from build123d import *

# Parameters (mm, degrees)
F1_DEPTH = 3


with BuildPart() as f1:
    # F0 (on Top) → F1 (new body)
    with BuildSketch(Plane.XY):
        with BuildLine():
            Line((-8, 15), (-0.625, 15))
            Line((-0.625, 15), (6.75, 15))
            Line((6.75, 15), (13.042543, 8.707457))
            Line((13.042543, 8.707457), (13.042543, 1.332457))
            Line((13.042543, 1.332457), (13.042543, -6.042543))
            Line((13.042543, -6.042543), (9.542543, -9.542543))
            ThreePointArc((9.542543, -9.542543), (8.864734, -11.345012), (9.773969, -13.042543))
            Line((9.773969, -13.042543), (14.542543, -13.042543))
            Line((14.542543, -13.042543), (14.542543, 16.5))
            Line((14.542543, 16.5), (-15, 16.5))
            Line((-15, 16.5), (-15, 11.5))
            ThreePointArc((-15, 11.5), (-13.25, 10.775126), (-11.5, 11.5))
            Line((-11.5, 11.5), (-8, 15))
        make_face()
    extrude(amount=F1_DEPTH)


solid = f1.part
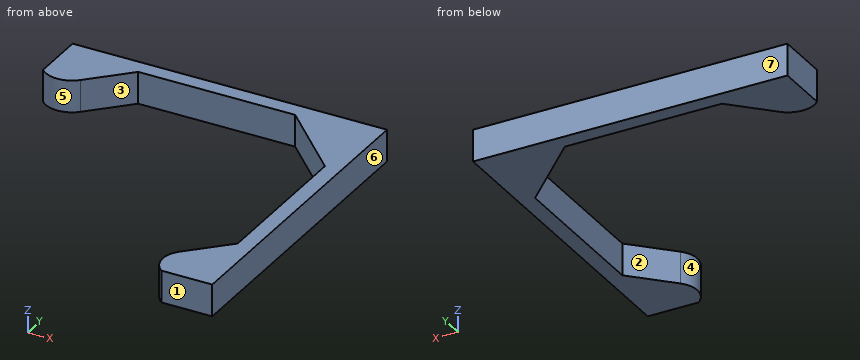
Geometry: final body of the model. Coordinates: model frame, mm. Face numbers are marked on the shaded views. A direction names the side the tool comes from. Coordinates: 2 decimals unless noted, no trailing zeros. Write each loop counter-clockwise with the first axis right and the second up, starting at its lowest first coordinate (ties: lowest second). Pieces come first, ordered by that corner, then holes. Notation, with made-up numbers: (9.5, 36) - (22.5, 36) arc R16 ccw to (22.5, 45) - close; hole circle Ø4 at (71.5, -18.75). An arc over 180 degrees is marked (long way). Return JSON: item names as keys, results as strings.
Item 1: Section query C-C (y = -3). Output: boundary loops of the cut face in (x, z), and give its area (3 significant figures).
Completed:
{"outline": "(13.04, 0) - (14.54, 0) - (14.54, 3) - (13.04, 3) - close", "area": "4.50 mm2"}
Item 2: Line query: L1, parallel to X at y = -11.25, z = 2.8; L2, parallel to X at y = 10.25, z = 0.8; L3, parallel to Y at x = 11, z = 2.1. Output: solid intervals per line, ascending.
Completed:
{"L1": "x = 8.86 to 14.54", "L2": "x = 11.5 to 14.54", "L3": "y = -13.04 to -8.09, 10.75 to 16.5"}
Item 3: Pull-direction query (X, two-part tool) for the marked faces 4, 5, 6 and 7; classes: +X half, -X half, draft (parallel to the pull), parting line (faces both ways), or undercut.
Completed:
{"face 4": "-X half", "face 5": "undercut", "face 6": "+X half", "face 7": "draft"}
Item 4: Section query B-B (x = 3). Output: boundary loops of the cut face in (y, z), and give its area (3 significant figures).
Completed:
{"outline": "(15, 0) - (16.5, 0) - (16.5, 3) - (15, 3) - close", "area": "4.50 mm2"}
Item 5: Reachability of the marked faces 1, 2 and 3 from +Z, -Z, +X, -X, +Y, -Y: full face, straight path, thin tool, end or side. Return the list, or none.
Completed:
{"face 1": "+Z, -Z, +X, -X, -Y", "face 2": "+Z, -Z, -X", "face 3": "+Z, -Z, -Y"}
Item 6: Section query A-A (z = 1.8). Output: boundary loops of the cut face in (x, y).
Completed:
{"outline": "(-15, 11.5) arc R2.47 ccw to (-11.5, 11.5) - (-8, 15) - (6.75, 15) - (13.04, 8.71) - (13.04, -6.04) - (9.54, -9.54) arc R2.33 ccw to (9.77, -13.04) - (14.54, -13.04) - (14.54, 16.5) - (-15, 16.5) - close"}
Item 7: Pin query (flat end, axial travel): pin 1 Ø0.9 at (x, z) = (2.5, 1) entering from -Y; pin 2 Ø1.5 at (y, z) = (-6.5, 2.5) entering from -X. Return the tip coordinate at first contact, or that it passes through.
Completed:
{"pin 1": "stops at y = 15", "pin 2": "stops at x = 11.84"}
